Here's the drawing with two shaded views (mm, measured from the low corner). I have some questions. A direction names the side the tool comes from. Round coordinates to 2 decimals unless told otherwise and drop trailing zeros. Order: outer loops, then holes, each group sorted by start corner. A loop starts at its lowest first (then second) coordinate and runs counter-clockwise, first axis right, second up.
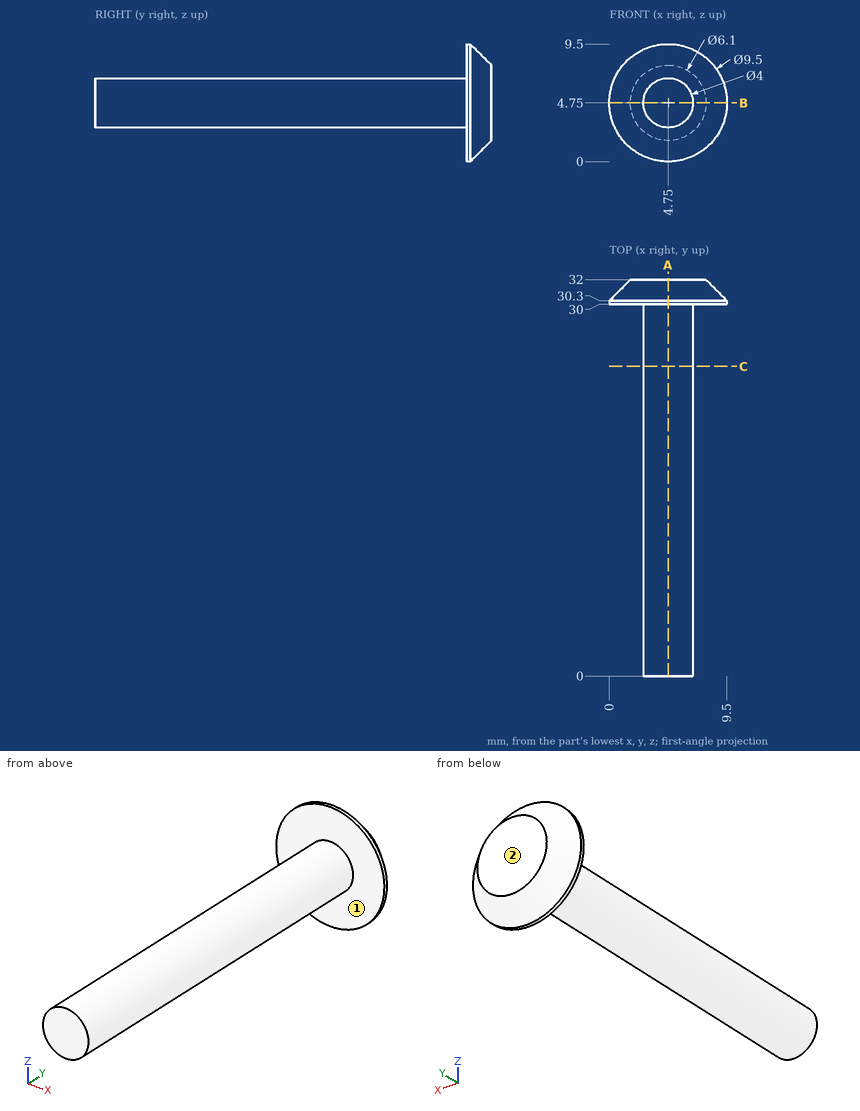
1. If we section it at A-A, the plane x = 4.75: Write out the boundary of the cut face in (y, z).
Evaluation:
outline: (0, 2.75) - (30, 2.75) - (30, 0) - (30.3, 0) - (32, 1.7) - (32, 7.8) - (30.3, 9.5) - (30, 9.5) - (30, 6.75) - (0, 6.75) - close
2. On a 3-axis mill with a long thin cutter (end or side, diameter ignored), from which of +Z, -Z, +X, -X, +Y, -Y can I reach the whole of each face in a straight line? I mean the marked faces 1 and 2. Say none if no direction works.
Evaluation:
face 1: -Y
face 2: +Z, -Z, +X, -X, +Y
3. I'm going to push flat-ended pins straight in: P1, Ø1.5, axis at x = 8, z = 6, coming from the +Y side; P2, Ø3, axis at x = 7, z = 1.5, coming from the -Y side; P3, Ø3, axis at y = 8.5, z = 5, coming from the -X side; P4, Ø5, axis at y = 4, z = 6, coming from the +X side. Where does each tip first touch, or does it pass through?
Evaluation:
P1: stops at y = 32
P2: stops at y = 30
P3: stops at x = 2.75
P4: stops at x = 6.75
4. If we section it at B-B, the plane z = 4.75: Write out the boundary of the cut face in (x, y).
Evaluation:
outline: (0, 30) - (2.75, 30) - (2.75, 0) - (6.75, 0) - (6.75, 30) - (9.5, 30) - (9.5, 30.3) - (7.8, 32) - (1.7, 32) - (0, 30.3) - close
5. If we section it at C-C, the plane y = 25: Write out the boundary of the cut face in (x, z).
Evaluation:
outline: circle Ø4 at (4.75, 4.75)
6. I need wall thicknesses on probe 1 along Y at (x, z) = (3.25, 6.25); probe 2 along X at (y, z) = (26.5, 4.75); probe 3 along Z at (x, y) = (6.5, 11). Which ranges of each line are inside material? Lowest first, please.
Evaluation:
probe 1: y = 30 to 32
probe 2: x = 2.75 to 6.75
probe 3: z = 3.78 to 5.72
